The model under review builds one solid part; all positions refer to its coordinate system, in mm. A direction names the side the tool comes from. Coordinates: 2 decimals unless noted, no trailing zeros. Write each loop counter-clockwise with the first axis right and the second up, starting at its lowest first coordinate (ties: lowest second). Pieces come first, ordered by that corner, then holes.
1) Mouldability with a two-part tool opening along Z and no side actions: class faces 4 (the cylindrical face through (0.546, -4.957, -0.651)), 5 (the cylindrical face through (-29.5, 4, 0)), 6 (the flat face through (0, 3, 0)), 7 (the flat face through (-42.5, 0, 0)) as released by +Z, released by -Z, zero draft, split by the parting line, or undercut.
2) Add section B-B, the plane x = 36.5. State the section outline as (y, z) points.
3) For P1, Ø3, axis at x = -9, y = 3, coming from the -Z side; P2, Ø4, axis at x = -20.5, y = -2.5, coming from the -Z side; P3, Ø1.2, axis at x = 8, z = 0, coming from the +Y side, all flat-tipped, find the tip position at first contact; note any pin that passes through.
4) Machinability: for faces 1 (the flat face through (42.5, 0, 0)), 2 (the cylindrical face through (39.76, 3.905, -0.867)), 3 (the cylindrical face through (29.5, 4, 0)), which of the approach directions +Z, -Z, +X, -X, +Y, -Y give a long, thin tool a straight path to every point of the face, cutting with its end or side? Answer none if there is none.
5) Add section C-C, the plane x = -21. State the section outline as (y, z) points, then the cut area to 3 significant figures.
6) Add section A-A, the plane z = 0. State the section outline as (x, y) points, then the cut area to 3 significant figures.
7) For line 1 (X direction, y = -3.5, z = -3.25); line 2 (X direction, y = 4.5, z = 0.5); line 3 (X direction, y = 3.25, z = 2.5), list the stretches that pass through material, from the lowest coordinate up.
from build123d import *

# Parameters (mm, degrees)
CHAMFER1_SIZE      = 1
SKETCH3_W          = 4
SKETCH3_H          = 4
CUT_EXTRUDE1_DEPTH = 5
CUT_EXTRUDE2_DEPTH = 10


with BuildPart() as part:
    # Sketch1 → Revolve1 (revolve)
    with BuildSketch(Plane.XY, mode=Mode.PRIVATE) as revolve1_sk:
        Polygon((-42.5, 0), (-42.5, 5), (-40.5, 5), (-40.5, 4), (-39, 4), (-39, 5), (39, 5), (39, 4), (40.5, 4), (40.5, 5), (42.5, 5), (42.5, 0), align=None)
    revolve(revolve1_sk.sketch.rotate(Axis((-47.151991765, 0, 0), (1, 0, 0)), 90), axis=Axis((-47.151991765, 0, 0), (1, 0, 0)))

    # Chamfer1
    chamfer1_edges = [part.edges().sort_by_distance(p)[0] for p in [
        (42.5, 0, -5),
        (-42.5, 0, -5),
    ]]
    chamfer(chamfer1_edges, length=CHAMFER1_SIZE)

    # Sketch3 → Cut-Extrude1 (cut)
    with BuildSketch(Plane(origin=(0, 0, 0), x_dir=(0, 0, -1), z_dir=(1, 0, 0))):
        with Locations((0, 5)):
            Rectangle(SKETCH3_W, SKETCH3_H)
    extrude(amount=-CUT_EXTRUDE1_DEPTH, mode=Mode.SUBTRACT)

    # Sketch4 → Cut-Extrude2 (cut)
    with BuildSketch(Plane(origin=(0, 3, 0), x_dir=(1, 0, 0), z_dir=(0, 1, 0))):
        with BuildLine():
            Line((27.5, -2), (0, -2))
            Line((0, -2), (-27.5, -2))
            ThreePointArc((-27.5, -2), (-29.5, 0), (-27.5, 2))
            Line((-27.5, 2), (0, 2))
            Line((0, 2), (27.5, 2))
            ThreePointArc((27.5, 2), (29.5, 0), (27.5, -2))
        make_face()
    extrude(amount=CUT_EXTRUDE2_DEPTH, mode=Mode.SUBTRACT)


solid = part.part
Geometry results:
1. face 4: split by the parting line
1. face 5: undercut
1. face 6: undercut
1. face 7: zero draft
2. outline: circle Ø10 at (0, 0)
3. P1: stops at z = -4.77
3. P2: stops at z = -4.97
3. P3: stops at y = 3
4. face 1: +Z, -Z, +X, +Y, -Y
4. face 2: none
4. face 3: +Y
5. outline: (3, -2) - (3, 2) - (4.58, 2) arc R5 ccw (long way) to (4.58, -2) - close
5. area: 71.1 mm2
6. outline: (-42.5, -4) - (-41.5, -5) - (-40.5, -5) - (-40.5, -4) - (-39, -4) - (-39, -5) - (39, -5) - (39, -4) - (40.5, -4) - (40.5, -5) - (41.5, -5) - (42.5, -4) - (42.5, 4) - (41.5, 5) - (40.5, 5) - (40.5, 4) - (39, 4) - (39, 5) - (29.5, 5) - (29.5, 3) - (-29.5, 3) - (-29.5, 5) - (-39, 5) - (-39, 4) - (-40.5, 4) - (-40.5, 5) - (-41.5, 5) - (-42.5, 4) - close
6. area: 724 mm2
7. line 1: x = -41.72 to -40.5, -39 to 39, 40.5 to 41.72
7. line 2: x = -41.97 to -40.5, -39 to -29.44, 29.44 to 39, 40.5 to 41.97
7. line 3: x = -42.4 to -40.5, -39 to 39, 40.5 to 42.4
